```python
from build123d import *

# Parameters (mm, degrees)
SKETCH1_W                        = 152.4
SKETCH1_H                        = 38.1
BOSS_EXTRUDE1_DEPTH              = 9.525
SKETCH5_W                        = 43.18
SKETCH5_H                        = 38.1
BOSS_EXTRUDE3_DEPTH              = 3.81
SKETCH3_W                        = 5.0419
SKETCH3_H                        = 3.81
F_3_8_CLEARANCE_HOLE1_AT_2_COUNT = 2
F_3_8_CLEARANCE_HOLE1_AT_2_PITCH = 25.4
SKETCH4_W                        = 51.528477944
SKETCH4_H                        = 38.1
BOSS_EXTRUDE2_DEPTH              = 8.89
F_3_8_CLEARANCE_HOLE3_D          = 10.0838
SKETCH10_R                       = 4.7625
CUT_EXTRUDE1_DEPTH               = 19.415


with BuildPart() as part:
    # Sketch1 → Boss-Extrude1 (new body)
    with BuildSketch(Plane.XY):
        Rectangle(SKETCH1_W, SKETCH1_H)
    extrude(amount=BOSS_EXTRUDE1_DEPTH)

    # Sketch5 → Boss-Extrude3 (add)
    with BuildSketch(Plane.XY.offset(9.525)):
        with Locations((54.61, 0)):
            Rectangle(SKETCH5_W, SKETCH5_H)
    extrude(amount=BOSS_EXTRUDE3_DEPTH)

    # Sketch3 → 3/8 Clearance Hole1 (revolve, cut)
    with BuildSketch(Plane(origin=(41.148, 0, 9.525), x_dir=(0, 1, 0), z_dir=(1, 0, 0))):
        with Locations((2.52095, 1.905)):
            Rectangle(SKETCH3_W, SKETCH3_H)
    f_3_8_clearance_hole1 = revolve(axis=Axis((41.148, 0, 3.175), (0, 0, 1)), mode=Mode.SUBTRACT)

    # 3/8 Clearance Hole1 at 2: 3/8 Clearance Hole1 ×2
    with Locations(*[(i * F_3_8_CLEARANCE_HOLE1_AT_2_PITCH, 0, 0) for i in range(1, F_3_8_CLEARANCE_HOLE1_AT_2_COUNT)]):
        add(f_3_8_clearance_hole1, mode=Mode.SUBTRACT)

    # Sketch4 → Boss-Extrude2 (add)
    with BuildSketch(Plane.XY.offset(9.525)):
        with Locations((-50.435761028, 0)):
            Rectangle(SKETCH4_W, SKETCH4_H)
    extrude(amount=BOSS_EXTRUDE2_DEPTH)

    # 3/8 Clearance Hole3 (through all)
    with Locations(Plane(origin=(0, 0, 0), x_dir=(-1, 0, 0), z_dir=(0, 0, -1))):
        with Locations((-66.548, 0), (-41.148, 0)):
            Hole(F_3_8_CLEARANCE_HOLE3_D / 2)

    # Sketch10 → Cut-Extrude1 (cut, through all)
    with BuildSketch(Plane.XY.offset(18.415)):
        with Locations((-60.452, 0)):
            Circle(SKETCH10_R)
    extrude(amount=-CUT_EXTRUDE1_DEPTH, mode=Mode.SUBTRACT)


solid = part.part
```
The listing builds one solid part. Answer for the finished solid, in the listing's coordinates (mm). A direction names the side the tool comes from. Give positions to 0.01 mm unless a question says otherwise; leave off trailing zeros. Write each loop counter-clockwise with the first axis right and the second up, starting at its lowest first coordinate (ties: lowest second). Pieces come first, ordered by that corner, then holes. Notation, with made-up numbers: (25.25, 74.5) -> (46.25, 74.5) arc R21 cw to (46.25, 100.5) -> close; hole circle Ø3 at (61, 29.5). An arc over 180 degrees is marked (long way). Write item = value, one per line. Start each with the question number.
1) Which of the six approach directions +Z, -Z, +X, -X, +Y, -Y give full straight-line access (tool end or side, diameter ignored) to faces 5 (the face through (4, 0, 9.525)), 6 (the face through (54, 0, 13.335)), 7 (the face through (-1, -19.05, 7))?
2) The part is cut by section D-D, the plane y = -15. Determine the outline of the cut face in (x, z) (3 decimals), and give its area (3 significant figures).
3) Determine the mould class of faces 1 (the face through (76.2, 0, 7)), 2 (the face through (-24.672, 0, 14)), 3 (the face through (-76.2, 0, 9)), 4 (the face through (-51, 0, 18.415)) for opening direction X: +X half, -X half, draft (parallel to the pull), parting line (faces both ways), or undercut.
4) Straight lines are drawn through the part: line 1 along X through (y, z) = (0.5, 13.25); line 2 along Y through (x, z) = (-60, 3.25); line 3 along Z through (x, y) = (22, 16.5) (3 decimals). For each, find the intervals that lie inside material, in ascending order.
5) The part is cut by section C-C, the plane z = 4.5. Count the separate pieces of the cut face and the enclosed holes in it, and give its area (3 significant figures).
6) The part is cut by section A-A, the plane y = 0. Determine the outline of the cut face in (x, z) (1 decimal).
7) Each of these flat-tipped pins is pushed along its axis until it touches: pin 1 (4 mm diameter, centred on y = 11.5, z = 15.5, fed in from +X); pin 2 (12.5 mm diameter, centred on x = -60.452, y = 0, fed in from -Z); pin 3 (11.5 mm diameter, centred on x = 60.5, y = -5, fed in from +Z) (3 decimals). Where does it stop, or does it pass through?
Solutions:
q1.face_5 = +Z, +Y, -Y
q1.face_6 = +Z, +X, +Y, -Y
q1.face_7 = +Z, -Z, +X, -X, -Y
q2.outline = (-76.2, 0) -> (76.2, 0) -> (76.2, 13.335) -> (33.02, 13.335) -> (33.02, 9.525) -> (-24.672, 9.525) -> (-24.672, 18.415) -> (-76.2, 18.415) -> close
q2.area = 2,070 mm²
q3.face_1 = +X half
q3.face_2 = undercut
q3.face_3 = -X half
q3.face_4 = draft
q4.line_1 = -76.2 to -65.19, -55.72 to -24.67, 33.02 to 36.13, 46.17 to 61.53, 71.57 to 76.2
q4.line_2 = -19.05 to -4.74, 4.74 to 19.05
q4.line_3 = 0 to 9.525
q5.separate_pieces = 1
q5.enclosed_holes = 3
q5.area = 5,580 mm²
q6.outline = (-76.2, 0) -> (-65.2, 0) -> (-65.2, 18.4) -> (-76.2, 18.4) -> close; (-55.7, 0) -> (36.1, 0) -> (36.1, 13.3) -> (33, 13.3) -> (33, 9.5) -> (-24.7, 9.5) -> (-24.7, 18.4) -> (-55.7, 18.4) -> close; (46.2, 0) -> (61.5, 0) -> (61.5, 13.3) -> (46.2, 13.3) -> close; (71.6, 0) -> (76.2, 0) -> (76.2, 13.3) -> (71.6, 13.3) -> close
q7.pin_1 = -24.67
q7.pin_2 = 0
q7.pin_3 = 13.335
